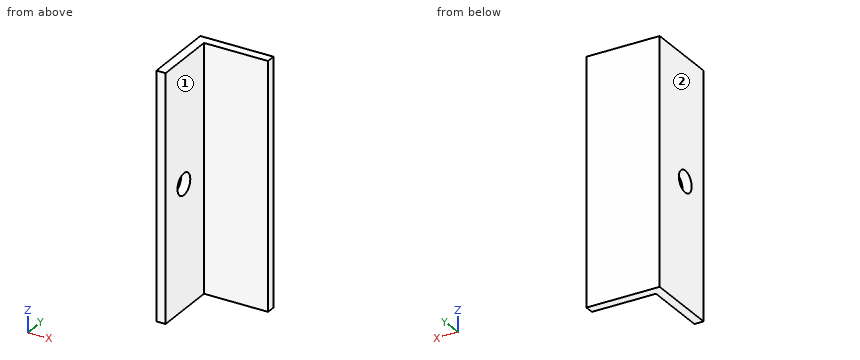
Autodesk Inventor part; units mm, degrees
ref_plane "YZ Plane" through (0, 0, 0) normal (1, 0, 0) x (0, 1, 0)
ref_plane "XZ Plane" through (0, 0, 0) normal (0, 1, 0) x (-1, 0, 0)
ref_plane "XY Plane" through (0, 0, 0) normal (0, 0, 1) x (1, 0, 0)
sketch "Szkic1" plane through (0, 0, 0) normal (0, 0, 1) x (1, 0, 0)
  line L0 (0, 0) -> (0, -12)
  line L1 (0, -12) -> (1.5, -12)
  line L2 (1.5, -12) -> (1.5, -1.5)
  line L3 (1.5, -1.5) -> (12, -1.5)
  line L4 (12, -1.5) -> (12, 0)
  line L5 (12, 0) -> (0, 0)
  dimension "d0" = 12
  dimension "d1" = 1.5
  dimension "d2" = 10.5
  dimension "d3" = 10.5
extrude "Wyciągnięcie proste1" add sketch "Szkic1" along normal mid plane 40
sketch "Szkic2" plane through (1.5, -12, 20) normal (1, 0, 0) x (0, 0, -1)
  line L0 (40, 0) -> (0, 0)
  line L1 (40, 0) -> (0, 0) construction
  line L2 (20, 0) -> (20, 5) construction
  point P0 (20, 12)
  dimension "d6" = 5
hole "Otwór1" at (1.5, -7, 0) direction (-1, 0, 0) diameter 3.5 end through all
properties part number "bepf_platforma_wspornik_poziomy" material "Aluminium 6061"
Design review of the part built by this model. Coordinates are the model's own, in mm. Face numbers are marked on the shaded views. A direction names the side the tool comes from. Coordinates: 2 decimals unless noted, no trailing zeros. Loops run counter-clockwise (first coordinate to the right, second up) from the corner with the lowest first, then second, coordinate; pieces in that order, holes last.
Q1. We need section A-A on y = -7. State the section outline as (x, z) points.
Reported:
outline: (0, -20) - (1.5, -20) - (1.5, -1.75) - (0, -1.75) - close; (0, 1.75) - (1.5, 1.75) - (1.5, 20) - (0, 20) - close
Q2. For pin 1 (2 mm diameter, centred on y = -6, z = -1.5, fed in from +X); pin 2 (1.5 mm diameter, centred on x = 9.5, z = 2, fed in from -Y), all flat-tipped, find the tip position at first contact; note any pin that passes through.
Reported:
pin 1: stops at x = 1.5
pin 2: stops at y = -1.5
Q3. We need section C-C on z = 5. State the section outline as (x, y) points, and give its area (4 significant figures).
Reported:
outline: (0, -12) - (1.5, -12) - (1.5, -1.5) - (12, -1.5) - (12, 0) - (0, 0) - close
area: 33.75 mm2
Q4. We need section B-B on z = 0. State the section outline as (x, y) points, and give its area (3 significant figures).
Reported:
outline: (0, -12) - (1.5, -12) - (1.5, -8.75) - (0, -8.75) - close; (0, -5.25) - (1.5, -5.25) - (1.5, -1.5) - (12, -1.5) - (12, 0) - (0, 0) - close
area: 28.5 mm2
Q5. Tool access review of the marked faces 1 and 2: name each direction out of +Z, -Z, +X, -X, +Y, -Y from which nothing blocks a thin tool from reaching the whole face with its end or side.
Reported:
face 1: +Z, -Z, +X, -Y
face 2: +Z, -Z, -X, +Y, -Y
Q6. To check wall thickness, follow line 1 (Z direction, x = 0.4, y = -7); line 2 (Y direction, x = 0.8, z = 0); line 3 (X direction, y = -5.5, z = -4). State the ranges of each line that lie inside material, in increasing order.
Reported:
line 1: z = -20 to -1.75, 1.75 to 20
line 2: y = -12 to -8.75, -5.25 to 0
line 3: x = 0 to 1.5
Q7. We need section D-D on x = 4.5. State the section outline as (y, z) points, and give its area (3 significant figures).
Reported:
outline: (-1.5, -20) - (0, -20) - (0, 20) - (-1.5, 20) - close
area: 60.0 mm2
